from build123d import *

# Parameters (mm, degrees)
SKETCH1_R                    = 400
BOSS_EXTRUDE1_DEPTH          = 20
SKETCH2_R                    = 25
CUT_EXTRUDE3_DEPTH           = 20
M12_TAPPED_HOLE1_D           = 10.2
M12_TAPPED_HOLE1_DEPTH       = 32.75
M12_TAPPED_HOLE1_CSINK_D     = 12.05
M12_TAPPED_HOLE1_CSINK_ANGLE = 90
M12_TAPPED_HOLE1_TIP         = 3.064389157


with BuildPart() as part:
    # Sketch1 → Boss-Extrude1 (new body)
    with BuildSketch(Plane(origin=(0, 0, 0), x_dir=(1, 0, 0), z_dir=(0, 1, 0))):
        Circle(SKETCH1_R)
    extrude(amount=BOSS_EXTRUDE1_DEPTH)

    # Sketch2 → Cut-Extrude3 (cut)
    with BuildSketch(Plane(origin=(0, 0, 0), x_dir=(1, 0, 0), z_dir=(0, 1, 0))):
        with Locations((102.698747746, 0)):
            Circle(SKETCH2_R)
        with Locations((202.698747746, 0)):
            Circle(SKETCH2_R)
        with Locations((302.698747746, 0)):
            Circle(SKETCH2_R)
        with Locations((-97.301252254, 0)):
            Circle(SKETCH2_R)
        with Locations((-197.301252254, 0)):
            Circle(SKETCH2_R)
        with Locations((-297.301252254, 0)):
            Circle(SKETCH2_R)
    extrude(amount=CUT_EXTRUDE3_DEPTH, mode=Mode.SUBTRACT)

    # M12 Tapped Hole1
    with Locations(Plane(origin=(0, 20, 0), x_dir=(1, 0, 0), z_dir=(0, 1, 0))):
        with Locations((0, 0)):
            CounterSinkHole(M12_TAPPED_HOLE1_D / 2, M12_TAPPED_HOLE1_CSINK_D / 2, depth=M12_TAPPED_HOLE1_DEPTH, counter_sink_angle=M12_TAPPED_HOLE1_CSINK_ANGLE)
            with Locations((0, 0, -(M12_TAPPED_HOLE1_DEPTH + M12_TAPPED_HOLE1_TIP / 2))):  # 118° drill point
                Cone(0, M12_TAPPED_HOLE1_D / 2, M12_TAPPED_HOLE1_TIP, mode=Mode.SUBTRACT)


solid = part.part
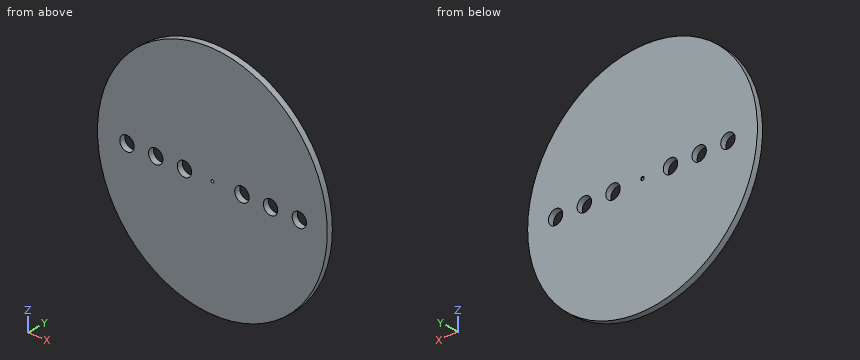
Work out the finished part from the listing and answer in its coordinate system (mm). Give positions to 0.01 mm unless a question says otherwise; leave off trailing zeros. Order: outer loops, then holes, each group sorted by start corner. A loop starts at its lowest first (then second) coordinate and runs counter-clockwise, first axis right, second up. Notation, with made-up numbers: (72, 84) -> (98, 84) arc R27 cw to (98, 102) -> close; hole circle Ø10 at (22, -29). An arc over 180 degrees is marked (long way). Answer as a JSON object with one key per item and string values. Group by question number.
1. Flat-ended cylindrical pins translate along their axes: pin 1 Ø4 at (x, y) = (-130.5, 7.5) entering from +Z; pin 2 Ø6 at (x, y) = (-241, 4) entering from -Z; pin 3 Ø3 at (y, z) = (6, -85) entering from -X. Find the tip coordinate at first contact, or state that the pin passes through.
2. Section B-B on x = -95 is taken. Determine the outline of the cut face in (y, z).
3. Section A-A on y = 11.5 is taken. Determine the outline of the cut face in (x, z), plus the area to 3 significant figures.
4. Consider line 1 along Z through (x, y) = (-87.5, 8.5); line 2 along Z through (x, y) = (102.5, 9.5); line 3 along Z through (x, y) = (-149.5, 8). Determine where each line is inside the solid, lowest interval first. Write a range as [from, to].
5. Section D-D on z = -96.5 is taken. Determine the outline of the cut face in (x, y).
6. Section C-C on x = 90 is taken. Determine the outline of the cut face in (y, z), plus the area to 3 significant figures.
Result sheet:
{
 "1": {"pin 1": "stops at z = 378.8", "pin 2": "stops at z = -321.49", "pin 3": "stops at x = -391.19"},
 "2": {"outline": "(0, -388.56) -> (20, -388.56) -> (20, -24.89) -> (0, -24.89) -> close; (0, 24.89) -> (20, 24.89) -> (20, 388.56) -> (0, 388.56) -> close"},
 "3": {"outline": "circle Ø800 at (0, 0); hole circle Ø50 at (-297.3, 0); hole circle Ø50 at (-197.3, 0); hole circle Ø50 at (-97.3, 0); hole circle Ø10.2 at (0, 0); hole circle Ø50 at (102.7, 0); hole circle Ø50 at (202.7, 0); hole circle Ø50 at (302.7, 0)", "area": "491,000 mm^2"},
 "4": {"line 1": "z = [-390.31, -23], [23, 390.31]", "line 2": "z = [-386.64, -25], [25, 386.64]", "line 3": "z = [-371.01, 371.01]"},
 "5": {"outline": "(-388.19, 0) -> (388.19, 0) -> (388.19, 20) -> (-388.19, 20) -> close"},
 "6": {"outline": "(0, -389.74) -> (20, -389.74) -> (20, -21.53) -> (0, -21.53) -> close; (0, 21.53) -> (20, 21.53) -> (20, 389.74) -> (0, 389.74) -> close", "area": "14,700 mm^2"}
}
